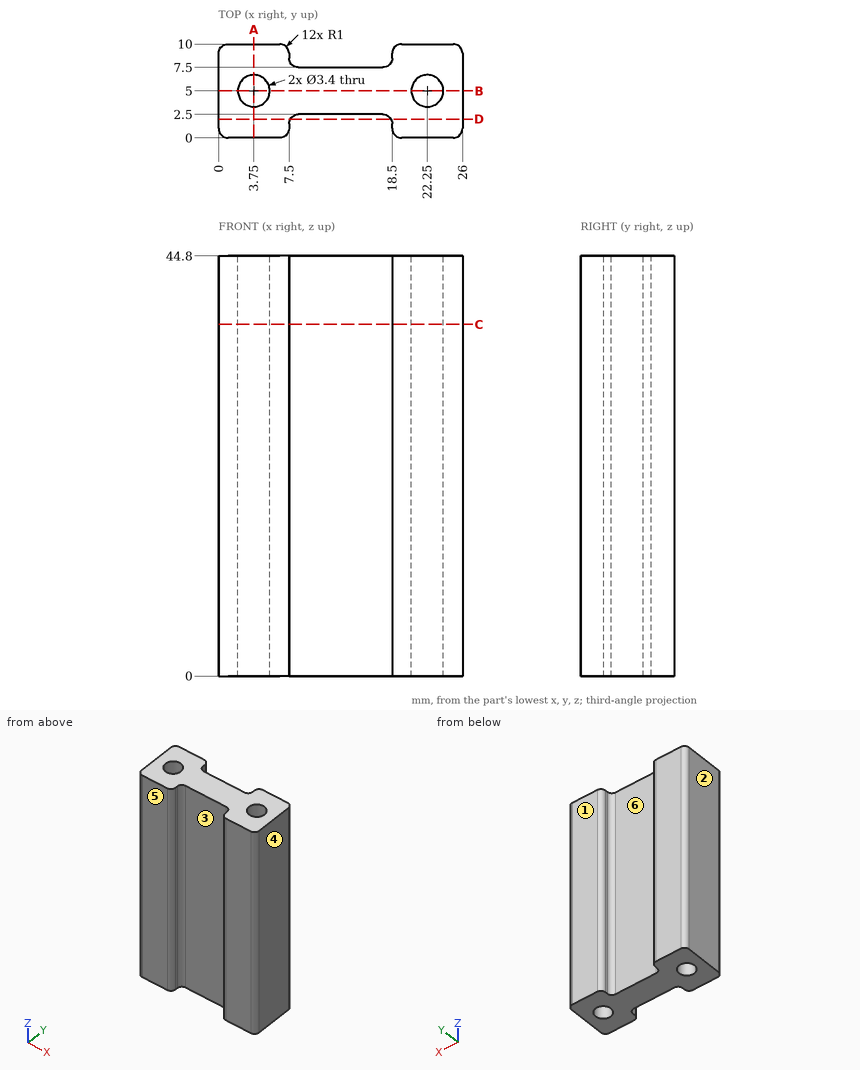
Can you work these out from the drawing? Everything is in mm from the part's minimum corner. A direction names the side the tool comes from. Round coordinates to 2 decimals unless told otherwise and drop trailing zeros. Loops run counter-clockwise (first coordinate to the right, second up) from the corner with the lowest first, then second, coordinate; pieces in that order, holes last. Notation, with made-up numbers: (18, 72) - (77, 72) arc R15 ccw to (77, 79) - close; hole circle Ø10 at (38, -26.5). An arc over 180 degrees is marked (long way). Write item = value, one per line. Start each with the question number.
(1) If I drill on probe 1 along X at (y, z) = (5, 24.5); probe 2 along Y at (x, z) = (22.25, 18); probe 3 along X at (y, z) = (1.5, 21), over which ranges is the centre line in solid material (lowest first)? Write a range as [from, to].
(2) For P1, Ø10, axis at x = 12, z = 33, coming from the -Y side; P2, Ø4.5, axis at x = 3.75, y = 5, coming from the -Z side; P3, Ø5, axis at x = 15.5, z = 12.5, coming from the -Y side; P4, Ø1, axis at x = 12.5, z = 26, coming from the -Y side, each with a flat end and sliding along its axis, tell me the tip position at first contact or that it passes through.
(3) If we section it at B-B (y = 5): Please give me the cut outline in (x, z), and give its area (3 significant figures).
(4) If we section it at D-D (y = 2): Please give me the cut outline in (x, z), and give its area (3 significant figures).
(5) If we mould it in two halves opening along X, with no side actions, what happens to the marked faces 1, 2, 3 and 4? For each: released by +X, released by -X, zero draft, split by the parting line, or undercut.
(6) If we section it at C-C (z = 37.5): Please give me the cut outline in (x, y).
(7) If we section it at A-A (x = 3.75): Please give me the cut outline in (y, z), and give its area (3 significant figures).
(8) For the marked faces 5 and 6, which set-ups out of +Z, -Z, +X, -X, +Y, -Y let a thin tool reach every point of the face, with its end or its side?
Ans:
q1.probe_1 = [0, 2.05], [5.45, 20.55], [23.95, 26]
q1.probe_2 = [0, 3.3], [6.7, 10]
q1.probe_3 = [0, 7.5], [18.5, 26]
q2.P1 = 0.13
q2.P2 = 0
q2.P3 = 2.37
q2.P4 = 2.5
q3.outline = (0, 0) - (2.05, 0) - (2.05, 44.8) - (0, 44.8) - close; (5.45, 0) - (20.55, 0) - (20.55, 44.8) - (5.45, 44.8) - close; (23.95, 0) - (26, 0) - (26, 44.8) - (23.95, 44.8) - close
q3.area = 860 mm²
q4.outline = (0, 0) - (7.63, 0) - (7.63, 44.8) - (0, 44.8) - close; (18.37, 0) - (26, 0) - (26, 44.8) - (18.37, 44.8) - close
q4.area = 684 mm²
q5.face_1 = zero draft
q5.face_2 = released by -X
q5.face_3 = undercut
q5.face_4 = released by +X
q6.outline = (0, 1) arc R1 ccw to (1, 0) - (6.5, 0) arc R1 ccw to (7.5, 1) - (7.5, 1.5) arc R1 cw to (8.5, 2.5) - (17.5, 2.5) arc R1 cw to (18.5, 1.5) - (18.5, 1) arc R1 ccw to (19.5, 0) - (25, 0) arc R1 ccw to (26, 1) - (26, 9) arc R1 ccw to (25, 10) - (19.5, 10) arc R1 ccw to (18.5, 9) - (18.5, 8.5) arc R1 cw to (17.5, 7.5) - (8.5, 7.5) arc R1 cw to (7.5, 8.5) - (7.5, 9) arc R1 ccw to (6.5, 10) - (1, 10) arc R1 ccw to (0, 9) - close; hole circle Ø3.4 at (3.75, 5); hole circle Ø3.4 at (22.25, 5)
q7.outline = (0, 0) - (3.3, 0) - (3.3, 44.8) - (0, 44.8) - close; (6.7, 0) - (10, 0) - (10, 44.8) - (6.7, 44.8) - close
q7.area = 296 mm²
q8.face_5 = +Z, -Z, +X, -X, -Y
q8.face_6 = +Z, -Z, +Y
